Source: CAD feature listing. Evaluate the final solid. Frame: model axes, mm. Coordinates: 2 decimals unless noted, no trailing zeros. Write each loop counter-clockwise with the first axis right and the second up, starting at its lowest first coordinate (ties: lowest second). Pieces come first, ordered by that corner, then holes. Notation, with made-up numbers: (42.25, 26.5) - (68.25, 26.5) arc R15 ccw to (68.25, 34.5) - close; hole circle Ø11 at (1, -35). An arc over 180 degrees is marked (long way). One line per item, written item: value.
Autodesk Fusion 360 part; units mm, degrees
sketch "Sketch1" plane through (0, 0, 0) normal (0, 0, 1) x (1, 0, 0)
  line L0 (0, 0) -> (0, 0)
  line L1 (9.525, 9.525) -> (9.525, 180.975)
  line L2 (0, 190.5) -> (0, 190.5)
  line L3 (-9.525, 180.975) -> (-9.525, 9.525)
  line L4 (0, 0) -> (0, 190.5) construction
  arc A0 (-9.525, 9.525) -> (0, 0) centre (0, 9.525) ccw
  arc A1 (0, 0) -> (9.525, 9.525) centre (0, 9.525) ccw
  arc A2 (0, 190.5) -> (-9.525, 180.975) centre (0, 180.975) ccw
  arc A3 (9.525, 180.975) -> (0, 190.5) centre (0, 180.975) ccw
  circle A4 centre (0, 182) radius 1.75
  circle A5 centre (0, 131.2) radius 1.75
  dimension "d1" = 190.5
  dimension "d2" = 19.05
  dimension "d3" = 9.525
  dimension "d4" = 9.525
  dimension "d5" = 9.525
  dimension "d6" = 9.525
  dimension "d7" = 3.5
  dimension "d8" = 3.5
  dimension "d9" = 50.8
extrude "Extrude1" add sketch "Sketch1" along normal blind 19.05
1) Contact query for flat-ended pins moving along their axis: P1, Ø4, axis at x = 0, y = 131.2, coming from the -Z side; P2, Ø8, axis at x = 5, z = 5, coming from the -Y side; P3, Ø4, axis at x = 6, z = 14, coming from the +Y side. Output: stop coordinate, or through.
Values found:
P1: z = 0
P2: y = 0.05
P3: y = 189.62
2) Section query A-A on x = 0. Output: boundary loops of the cut face in (y, z).
Values found:
outline: (0, 0) - (129.45, 0) - (129.45, 19.05) - (0, 19.05) - close; (132.95, 0) - (180.25, 0) - (180.25, 19.05) - (132.95, 19.05) - close; (183.75, 0) - (190.5, 0) - (190.5, 19.05) - (183.75, 19.05) - close
3) Draft query along X for faces 1 (the flat face through (0, 97, 19.05)), 2 (the cylindrical face through (-0.209, 190.498, 9.392)), 3 (the cylindrical face through (0.81, 132.75, 9.39)), 4 (the cylindrical face through (0.81, 183.55, 9.39)). Return one class per face: released by +X, released by -X, zero draft, split by the parting line, or undercut.
Values found:
face 1: zero draft
face 2: split by the parting line
face 3: undercut
face 4: undercut
4) Section query C-C on z = 10.5. Output: boundary loops of the cut face in (x, y) (3 decimals).
Values found:
outline: (-9.525, 9.525) arc R9.525 ccw to (9.525, 9.525) - (9.525, 180.975) arc R9.525 ccw to (-9.525, 180.975) - close; hole circle Ø3.5 at (0, 131.2); hole circle Ø3.5 at (0, 182)
5) Section query B-B on y = 131.2. Output: boundary loops of the cut face in (x, z) (3 decimals), then the cut area to 3 significant figures.
Values found:
outline: (-9.525, 0) - (-1.75, 0) - (-1.75, 19.05) - (-9.525, 19.05) - close; (1.75, 0) - (9.525, 0) - (9.525, 19.05) - (1.75, 19.05) - close
area: 296 mm2
6) Material intervals for line 1 (Y direction, x = 0, z = 7.25); line 2 (X direction, y = 131.2, z = 5) (3 decimals); line 3 (X direction, y = 9, z = 17), sorted ascending.
Values found:
line 1: 0 to 129.45, 132.95 to 180.25, 183.75 to 190.5
line 2: -9.525 to -1.75, 1.75 to 9.525
line 3: -9.51 to 9.51
